Verification items for this drawing (mm, ordinates from the low corner). Round coordinates to 2 decimals unless told otherwise and drop trailing zeros. Order: outer loops, then holes, each group sorted by start corner. A loop starts at its lowest first (then second) coordinate and runs counter-clockwise, first axis right, second up. Notation, with made-up numbers: (82, 77.5) -> (116, 77.5) arc R23 cw to (116, 92.5) -> close; hole circle Ø2 at (23.5, -20.75). An arc over 180 degrees is marked (long way). Use a Markdown table: item, result. Add a question column.
Item 1: Gauge pin test, flat end, axial feed: pin 1 Ø1.5 at (x, z) = (10, 20) entering from -Y. Record the tip position at first contact, or that the pin passes through.
Item 2: Material ranges on probe 1 along Z at (x, y) = (6.5, 1.45), recorded low to high. Write a range as [from, to].
Item 3: Sectioned sample at C-C, the plane y = 0.8. Record the cut outline in (x, z).
Item 4: Sectioned sample at B-B, the plane x = 7. Record the cut outline in (y, z), and give its area (3 significant figures).
Item 5: Sectioned sample at A-A, the plane z = 18. Record the cut outline in (x, y), and give its area (3 significant figures).
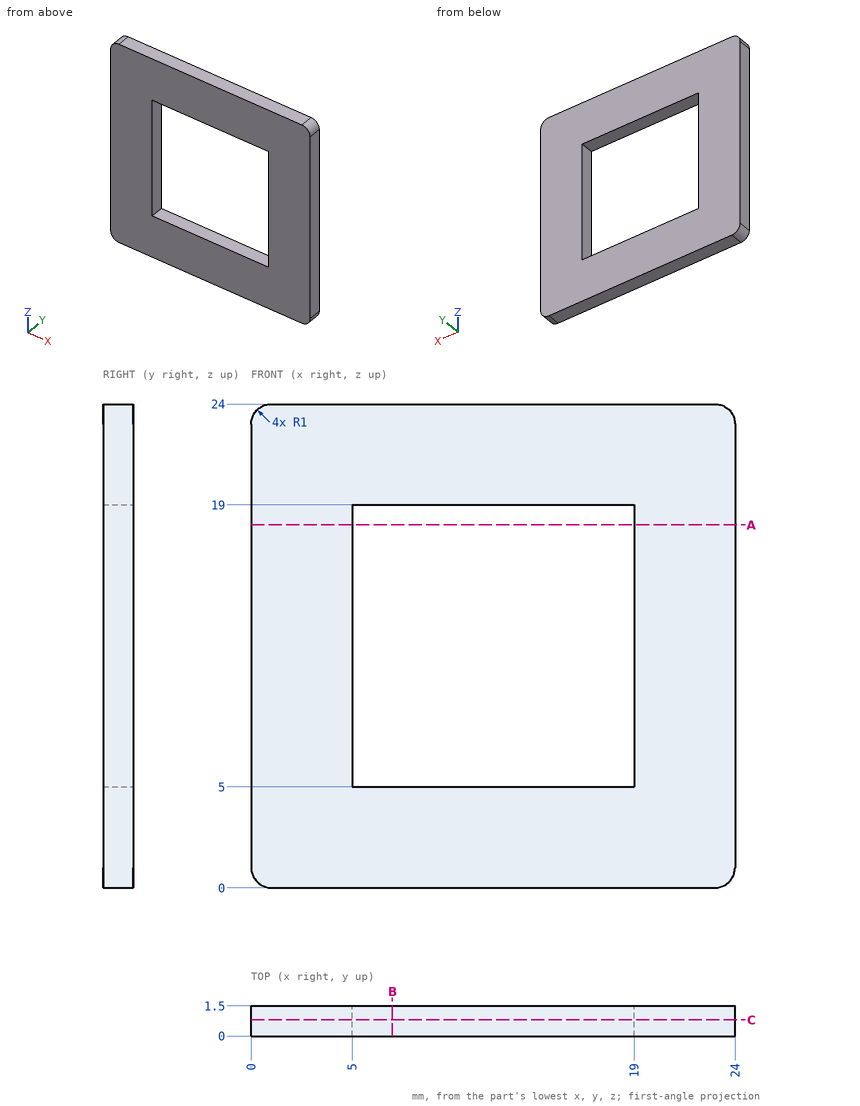
Found:
| question | item | result |
|---|---|---|
| 1 | pin 1 | stops at y = 0 |
| 2 | probe 1 | z = [0, 5], [19, 24] |
| 3 | outline | (0, 1) arc R1 ccw to (1, 0) -> (23, 0) arc R1 ccw to (24, 1) -> (24, 23) arc R1 ccw to (23, 24) -> (1, 24) arc R1 ccw to (0, 23) -> close; hole (5, 5) -> (19, 5) -> (19, 19) -> (5, 19) -> close |
| 4 | outline | (0, 0) -> (1.5, 0) -> (1.5, 5) -> (0, 5) -> close; (0, 19) -> (1.5, 19) -> (1.5, 24) -> (0, 24) -> close |
| 4 | area | 15.0 mm2 |
| 5 | outline | (0, 0) -> (5, 0) -> (5, 1.5) -> (0, 1.5) -> close; (19, 0) -> (24, 0) -> (24, 1.5) -> (19, 1.5) -> close |
| 5 | area | 15.0 mm2 |
